Autodesk Inventor part; units mm, degrees
ref_plane "YZ Plane" through (0, 0, 0) normal (1, 0, 0) x (0, 1, 0)
ref_plane "XZ Plane" through (0, 0, 0) normal (0, 1, 0) x (-1, 0, 0)
ref_plane "XY Plane" through (0, 0, 0) normal (0, 0, 1) x (1, 0, 0)
sketch "Sketch1" plane through (0, 0, 0) normal (0, 0, 1) x (1, 0, 0)
  line L0 (-99.06, 19.05) -> (469.9, 19.05)
  line L1 (469.9, 19.05) -> (469.9, -38.1)
  line L2 (469.9, -38.1) -> (-99.06, -38.1)
  line L3 (-99.06, -38.1) -> (-99.06, 19.05)
  circle A0 centre (-58.42, -9.525) radius 13
  circle A1 centre (41.716, -9.525) radius 13
  circle A2 centre (131.092, -9.525) radius 16
  circle A3 centre (429.26, -9.525) radius 13
  circle A4 centre (329.124, -9.525) radius 13
  circle A5 centre (239.748, -9.525) radius 16
  point P0 (0, 0)
  dimension "d4" = 26
  dimension "d6" = 26
  dimension "d8" = 32
  dimension "d10" = 26
  dimension "d12" = 26
  dimension "d14" = 32
  dimension "d16" = 568.96
  dimension "d17" = 57.15
  dimension "d18" = 40.64
  dimension "d19" = 140.776
  dimension "d20" = 230.152
  dimension "d21" = 230.152
  dimension "d22" = 40.64
  dimension "d23" = 140.776
extrude "Extrusion1" add sketch "Sketch1" along normal blind 9.525
properties part number "side"
Geometry: final body of the model. Coordinates: model frame, mm. Coordinates: 2 decimals unless noted, no trailing zeros. Order: outer loops, then holes, each group sorted by start corner. A loop starts at its lowest first (then second) coordinate and runs counter-clockwise, first axis right, second up.
1) Section C-C (z = 7). Return loops of the section in (x, y) (3 decimals), then the cut area to 3 significant figures.
Result sheet:
outline: (-99.06, -38.1) - (469.9, -38.1) - (469.9, 19.05) - (-99.06, 19.05) - close; hole circle Ø26 at (-58.42, -9.525); hole circle Ø26 at (41.716, -9.525); hole circle Ø32 at (131.092, -9.525); hole circle Ø32 at (239.748, -9.525); hole circle Ø26 at (329.124, -9.525); hole circle Ø26 at (429.26, -9.525)
area: 28,800 mm2
2) Draft query along Y for faces 1 (the cylindrical face through (416.273, -10.097, 4.696)), 2 (the flat face through (469.9, -9, 5)), 3 (the flat face through (189, -38.1, 5)). Return one class per face: released by +Y, released by -Y, zero draft, split by the parting line, or undercut.
Result sheet:
face 1: undercut
face 2: zero draft
face 3: released by -Y
3) Section A-A (x = 429.26). Return loops of the section in (y, z) (3 decimals).
Result sheet:
outline: (-38.1, 0) - (-22.525, 0) - (-22.525, 9.525) - (-38.1, 9.525) - close; (3.475, 0) - (19.05, 0) - (19.05, 9.525) - (3.475, 9.525) - close
4) Section D-D (x = 243). Return loops of the section in (y, z) (3 decimals).
Result sheet:
outline: (-38.1, 0) - (-25.191, 0) - (-25.191, 9.525) - (-38.1, 9.525) - close; (6.141, 0) - (19.05, 0) - (19.05, 9.525) - (6.141, 9.525) - close
5) Ray query, probe 1 along Y at (x, z) = (429.26, 7) (3 decimals); probe 2 along X at (y, z) = (-24, 9.25); probe 3 along Y at (x, z) = (49.5, 7). Return the intervals inside material, ascending.
Result sheet:
probe 1: y = -38.1 to -22.525, 3.475 to 19.05
probe 2: x = -99.06 to 124.27, 137.91 to 232.93, 246.57 to 469.9
probe 3: y = -38.1 to -19.94, 0.89 to 19.05
6) First-contact query: P1, Ø19, axis at x = 131.092, y = -9.525, coming from the -Z side. Flat tip, straight axial feed; report the tip coordinate or a pass-through.
Result sheet:
P1: passes through
7) Section B-B (y = -16.5). Return loops of the section in (x, z) (3 decimals), then the cut area to 3 significant figures.
Result sheet:
outline: (-99.06, 0) - (-69.39, 0) - (-69.39, 9.525) - (-99.06, 9.525) - close; (-47.45, 0) - (30.746, 0) - (30.746, 9.525) - (-47.45, 9.525) - close; (52.686, 0) - (116.692, 0) - (116.692, 9.525) - (52.686, 9.525) - close; (145.492, 0) - (225.348, 0) - (225.348, 9.525) - (145.492, 9.525) - close; (254.148, 0) - (318.154, 0) - (318.154, 9.525) - (254.148, 9.525) - close; (340.094, 0) - (418.29, 0) - (418.29, 9.525) - (340.094, 9.525) - close; (440.23, 0) - (469.9, 0) - (469.9, 9.525) - (440.23, 9.525) - close
area: 4,030 mm2
